from build123d import *

# Parameters (mm, degrees)
ESQUISSE1_R                = 38.1
BOSS_EXTRU_1_DEPTH         = 23.7
ESQUISSE2_R                = 12.7
ENL_V_MAT_EXTRU_1_DEPTH    = 7.3
ESQUISSE3_R                = 11.1125
ENL_V_MAT_EXTRU_2_DEPTH    = 2.7
ESQUISSE4_R                = 25.4
ENL_V_MAT_EXTRU_3_DEPTH    = 56.59595309
ESQUISSE6_OUTSIDE_W        = 100.268
ESQUISSE6_OUTSIDE_H        = 100.268
ESQUISSE6_OUTSIDE_R        = 34.925
ENL_V_MAT_EXTRU_4_DEPTH    = 2
R_P_TITION_LIN_AIRE1_COUNT = 4
R_P_TITION_LIN_AIRE1_PITCH = 4


with BuildPart() as part:
    # Esquisse1 → Boss.-Extru.1 (new body)
    with BuildSketch(Plane.XY):
        Circle(ESQUISSE1_R)
    extrude(amount=BOSS_EXTRU_1_DEPTH)

    # Esquisse2 → Enlèv. mat.-Extru.1 (cut)
    with BuildSketch(Plane(origin=(0, 0, 0), x_dir=(-1, 0, 0), z_dir=(0, 0, -1))):
        Circle(ESQUISSE2_R)
    extrude(amount=-ENL_V_MAT_EXTRU_1_DEPTH, mode=Mode.SUBTRACT)

    # Esquisse3 → Enlèv. mat.-Extru.2 (cut)
    with BuildSketch(Plane(origin=(0, 0, 7.3), x_dir=(-1, 0, 0), z_dir=(0, 0, -1))):
        Circle(ESQUISSE3_R)
    extrude(amount=-ENL_V_MAT_EXTRU_2_DEPTH, mode=Mode.SUBTRACT)

    # Esquisse4 → Enlèv. mat.-Extru.3 (cut, through all)
    with BuildSketch(Plane(origin=(0, 0, 10), x_dir=(-1, 0, 0), z_dir=(0, 0, -1))):
        Circle(ESQUISSE4_R)
    extrude(amount=-ENL_V_MAT_EXTRU_3_DEPTH, mode=Mode.SUBTRACT)

    # Esquisse6 outside → Enlèv. mat.-Extru.4 (cut)
    with BuildSketch(Plane(origin=(0, 0, 7.3), x_dir=(-1, 0, 0), z_dir=(0, 0, -1))):
        Rectangle(ESQUISSE6_OUTSIDE_W, ESQUISSE6_OUTSIDE_H)
        Circle(ESQUISSE6_OUTSIDE_R, mode=Mode.SUBTRACT)
    enl_v_mat_extru_4 = extrude(amount=-ENL_V_MAT_EXTRU_4_DEPTH, mode=Mode.SUBTRACT)

    # Répétition linéaire1: Enlèv. mat.-Extru.4 ×4
    with Locations(*[(0, 0, i * R_P_TITION_LIN_AIRE1_PITCH) for i in range(1, R_P_TITION_LIN_AIRE1_COUNT)]):
        add(enl_v_mat_extru_4, mode=Mode.SUBTRACT)


solid = part.part
CAD build for the part. Positions are in the model's coordinates, mm. A direction names the side the tool comes from. Round coordinates to 2 decimals unless told otherwise and drop trailing zeros. Write each loop counter-clockwise with the first axis right and the second up, starting at its lowest first coordinate (ties: lowest second). Pieces come first, ordered by that corner, then holes. Notation, with made-up numbers: M 84.25,28.5 L 100.25,28.5 A26 cw 100.25,49.5 Z; hole C -24,24.5 d4. An arc over 180 degrees is marked long. Use a Markdown table: item, result. Add a question column.
1. Slice it at A-A on z = 4. Give the cut face in (x, y), then the cut area to 3 significant figures.
2. 3-axis set-ups, long thin cutter, end or side, ignore diameter. For faces 1 (the face through (27.715, -21.251, 8.286)), 2 (the face through (5.506, -24.796, 16.754)), 3 (the face through (-30.235, -23.183, 22.483)): which of +Z, -Z, +X, -X, +Y, -Y reach the whole face in a straight line?
3. Flat gauge pins, fed straight in: P1, Ø8, axis at x = -22, z = 13.5, coming from the -Y side; P2, Ø8, axis at y = -20, z = 10.5, coming from the -X side; P3, Ø23, axis at x = 0, y = 0, coming from the -Z side; P4, Ø1, axis at x = -8.5, y = -17, coming from the -Z side. Where does each tip first touch, or does it go through?
4. Pull direction Z, two halves, no side cores. Call faces 4 (the face through (-11, -5, 10)), 5 (the face through (2.75, -12.4, 3.6)), 6 (the face through (16, 1, 0)), 7 (the face through (-17, -31, 19.3)): released by +Z, released by -Z, zero draft, split by the parting line, or undercut.
5. Drill centre lines: probe 1 along Z at (x, y) = (-32.5, -19); probe 2 along Y at (x, z) = (0, 8.55) (1 decimal); probe 3 along Y at (x, z) = (0, 15). Where is each one in solid material? Low to high.
Reply:
| question | item | result |
|---|---|---|
| 1 | outline | C 0,0 d76.2; hole C 0,0 d25.4 |
| 1 | area | 4,050 mm^2 |
| 2 | face 1 | none |
| 2 | face 2 | +Z |
| 2 | face 3 | +Z, -Z |
| 3 | P1 | stops at y = -33.58 |
| 3 | P2 | stops at x = -34.58 |
| 3 | P3 | stops at z = 7.3 |
| 3 | P4 | stops at z = 0 |
| 4 | face 4 | released by +Z |
| 4 | face 5 | zero draft |
| 4 | face 6 | released by -Z |
| 4 | face 7 | undercut |
| 5 | probe 1 | z = 0 to 7.3, 9.3 to 11.3, 13.3 to 15.3, 17.3 to 19.3, 21.3 to 23.7 |
| 5 | probe 2 | y = -34.9 to -11.1, 11.1 to 34.9 |
| 5 | probe 3 | y = -38.1 to -25.4, 25.4 to 38.1 |
